from build123d import *

# Parameters (mm, degrees)
SKETCH1_R           = 0.9
BOSS_EXTRUDE1_DEPTH = 2.85
SKETCH1_3_R         = 11
SKETCH1_3_R_2       = 8.5
BOSS_EXTRUDE2_DEPTH = 1
FILLET1_R           = 1


with BuildPart() as part:
    # Sketch1 → Boss-Extrude1 (new body)
    # profile 1 of 4: a face of its own
    with BuildSketch(Plane(origin=(0, 0, 0), x_dir=(1, 0, 0), z_dir=(0, 1, 0))):
        with BuildLine():
            ThreePointArc((-8.748809449, -6.667708244), (-9.526279442, -5.5), (-10.148809449, -4.242837113))
            Line((-10.148809449, -4.242837113), (-13.633676971, -6.254826316))
            ThreePointArc((-13.633676971, -6.254826316), (-13.326581008, -6.884928368), (-12.990383551, -7.49999568))
            ThreePointArc((-12.990383551, -7.49999568), (-12.625816068, -8.098689315), (-12.233676971, -8.679697446))
            Line((-12.233676971, -8.679697446), (-8.748809449, -6.667708244))
        make_face()
        with Locations(Location((-10.825317547, -6.25, 0), (0, 0, 90))):
            Circle(SKETCH1_R, mode=Mode.SUBTRACT)
    # profile 2 of 4: a face of its own
    with BuildSketch(Plane(origin=(0, 0, 0), x_dir=(1, 0, 0), z_dir=(0, 1, 0))):
        with BuildLine():
            ThreePointArc((-1.4, 10.910545358), (-0.701427497, 10.97761356), (0, 11))
            Line((0, 11), (0, 11.6))
            ThreePointArc((0, 11.6), (-0.9, 12.5), (0, 13.4))
            Line((0, 13.4), (0, 15))
            ThreePointArc((0, 15), (-0.700765142, 14.983621999), (-1.4, 14.934523762))
            Line((-1.4, 14.934523762), (-1.4, 10.910545358))
        make_face()
    # profile 3 of 4: a face of its own
    with BuildSketch(Plane(origin=(0, 0, 0), x_dir=(1, 0, 0), z_dir=(0, 1, 0))):
        with BuildLine():
            Line((0, 11.6), (0, 11))
            ThreePointArc((0, 11), (0.701427497, 10.97761356), (1.4, 10.910545358))
            Line((1.4, 10.910545358), (1.4, 14.934523762))
            ThreePointArc((1.4, 14.934523762), (0.700765142, 14.983621999), (0, 15))
            Line((0, 15), (0, 13.4))
            ThreePointArc((0, 13.4), (0.636396103, 13.136396103), (0.9, 12.5))
            ThreePointArc((0.9, 12.5), (0.636396103, 11.863603897), (0, 11.6))
        make_face()
    # profile 4 of 4: a face of its own
    with BuildSketch(Plane(origin=(0, 0, 0), x_dir=(1, 0, 0), z_dir=(0, 1, 0))):
        with BuildLine():
            Line((13.633676971, -6.254826316), (10.148809449, -4.242837113))
            ThreePointArc((10.148809449, -4.242837113), (9.526279442, -5.5), (8.748809449, -6.667708244))
            Line((8.748809449, -6.667708244), (12.233676971, -8.679697446))
            ThreePointArc((12.233676971, -8.679697446), (12.625814755, -8.098691362), (12.990381119, -7.499999892))
            ThreePointArc((12.990381119, -7.499999892), (13.326579892, -6.884930529), (13.633676971, -6.254826316))
        make_face()
        with Locations(Location((10.825317547, -6.25, 0), (0, 0, 90))):
            Circle(SKETCH1_R, mode=Mode.SUBTRACT)
    extrude(amount=BOSS_EXTRUDE1_DEPTH)

    # Sketch1_3 → Boss-Extrude2 (add)
    with BuildSketch(Plane(origin=(0, 0, 0), x_dir=(1, 0, 0), z_dir=(0, 1, 0))):
        Circle(SKETCH1_3_R)
        with Locations(Location((0, 0, 0), (0, 0, 270))):
            Circle(SKETCH1_3_R_2, mode=Mode.SUBTRACT)
    extrude(amount=BOSS_EXTRUDE2_DEPTH)

    # Fillet1
    fillet1_edges = [part.edges().sort_by_distance(p)[0] for p in [
        (-10.148809449, 0.5, 4.242837113),
        (-8.748809449, 0.5, 6.667708244),
        (-1.4, 0.5, -10.910545358),
        (1.4, 0.5, -10.910545358),
        (10.148809449, 0.5, 4.242837113),
        (8.748809449, 0.5, 6.667708244),
    ]]
    fillet(fillet1_edges, radius=FILLET1_R)


solid = part.part
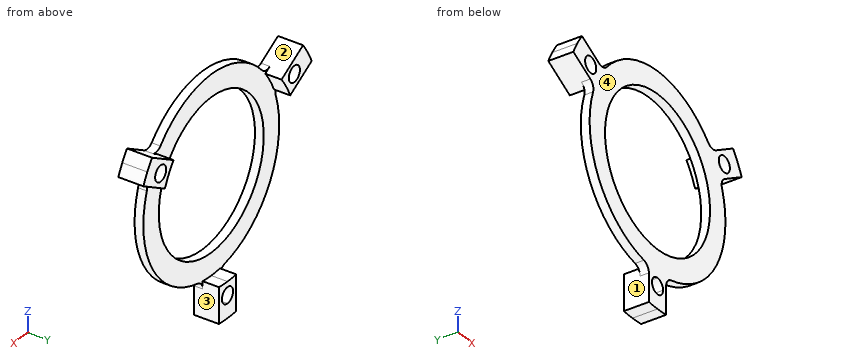
Source: CAD feature listing. Evaluate the final solid. Frame: model axes, mm. Face numbers are marked on the shaded views. A direction names the side the tool comes from. Coordinates: 2 decimals unless noted, no trailing zeros. Order: outer loops, then holes, each group sorted by start corner. A loop starts at its lowest first (then second) coordinate and runs counter-clockwise, first axis right, second up.
Item 1: Cut plane B-B (z = 0). Return loops of the section in (x, y).
Output values:
outline: (-11, 0) - (-8.5, 0) - (-8.5, 1) - (-11, 1) - close; (8.5, 0) - (11, 0) - (11, 1) - (8.5, 1) - close
Item 2: Cut plane A-A (y = 1.5). Return loops of the section in (x, z), plus the area to 3 significant figures.
Output values:
outline: (-13.63, 6.25) - (-10.15, 4.24) arc R11 cw to (-8.75, 6.67) - (-12.23, 8.68) arc R15 ccw to start; (-1.4, -14.93) arc R15 ccw to (1.4, -14.93) - (1.4, -10.91) arc R11 cw to (-1.4, -10.91) - close; (8.75, 6.67) arc R11 cw to (10.15, 4.24) - (13.63, 6.25) arc R15 ccw to (12.23, 8.68) - close; hole circle Ø1.8 at (-10.83, 6.25); hole circle Ø1.8 at (0, -12.5); hole circle Ø1.8 at (10.83, 6.25)
area: 26.0 mm2
Item 3: First-contact query: P1, Ø1.4, axis at y = 2, z = -13, coming from the -X side; P2, Ø0.9, axis at y = 2, z = -13.5, coming from the +X side; P3, Ø2, axis at x = 7, z = -5.5, coming from the +Y side; P4, Ø10, axis at x = 0, z = 0, coming from the +Y side. Flat tips, straight axial feed; report the tip coordinate or a pass-through.
Output values:
P1: stops at x = -1.4
P2: stops at x = 1.4
P3: stops at y = 1
P4: passes through
Item 4: Material intervals for line 1 (X direction, y = 0.3, z = 0); line 2 (Z direction, x = -5, y = 0.45); line 3 (Z direction, x = 7, y = 0.75), sorted ascending.
Output values:
line 1: x = -11 to -8.5, 8.5 to 11
line 2: z = -9.8 to -6.87, 6.87 to 9.8
line 3: z = -8.49 to -4.82, 4.82 to 8.49
Item 5: Pull-direction query (Y, two-part tool) for the marked faces 3 and 4; classes: pulls with the +Y half, pulls with the -Y half, needs draft (parallel to the pull), parting line crosses it, or undercut.
Output values:
face 3: needs draft
face 4: pulls with the -Y half
Item 6: Cut plane C-C (x = -4.5). Return loops of the section in (y, z), plus the area to 3 significant figures.
Output values:
outline: (0, -10.04) - (1, -10.04) - (1, -7.21) - (0, -7.21) - close; (0, 7.21) - (1, 7.21) - (1, 10.04) - (0, 10.04) - close
area: 5.65 mm2
Item 7: Set-up query: the marked faces 1 and 2. Return all of +Z, -Z, +X, -X, +Y, -Y with unobstructed straight access to the full face (end or side cutting, diameter ignored); none if empty.
Output values:
face 1: -Z, -X, +Y
face 2: +Z, +Y
